from build123d import *

# Parameters (mm, degrees)
F0_R     = 10.5
F0_R_2   = 9.5
F1_DEPTH = 10
F0_W     = 35
F0_H     = 35
F2_DEPTH = 1
F3_R     = 0.4
F4_R     = 0.5


with BuildPart() as f1:
    # F0 (on Top) → F1 (new body)
    with BuildSketch(Plane.XY):
        Circle(F0_R)
        Circle(F0_R_2, mode=Mode.SUBTRACT)
    extrude(amount=F1_DEPTH)

    # F0 (on Top) → F2 (join)
    with BuildSketch(Plane.XY):
        Rectangle(F0_W, F0_H)
        Circle(F0_R, mode=Mode.SUBTRACT)
        Circle(F0_R)
        Circle(F0_R_2, mode=Mode.SUBTRACT)
        Circle(F0_R_2)
    extrude(amount=-F2_DEPTH)

    # F3
    f3_edges = [f1.edges().sort_by_distance(p)[0] for p in [
        (-17.5, 0, -1),
        (0, 17.5, -1),
        (17.5, 0, -1),
        (0, -17.5, -1),
    ]]
    fillet(f3_edges, radius=F3_R)

    # F4
    f4_edges = [f1.edges().sort_by_distance(p)[0] for p in [
        (-9.5, 0, 10),
    ]]
    fillet(f4_edges, radius=F4_R)


solid = f1.part
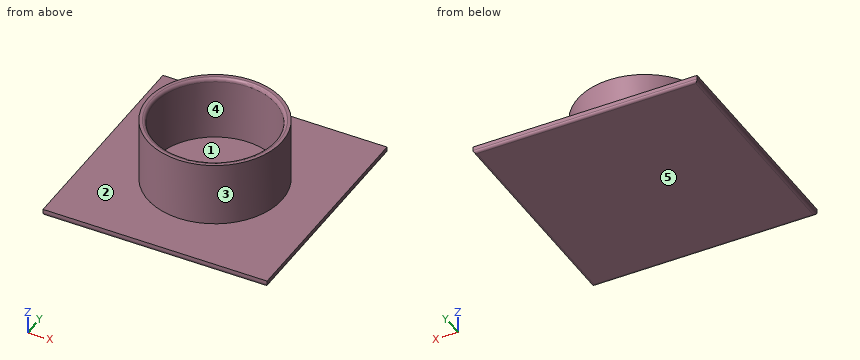
Check sheet for the modelled part. Datum: model origin and axes. Units: mm. Face numbers are marked on the shaded views. A direction names the side the tool comes from. Give positions to 0.01 mm unless a question says otherwise; leave off trailing zeros. Order: outer loops, then holes, each group sorted by start corner. A loop starts at its lowest first (then second) coordinate and runs counter-clockwise, first axis right, second up. Notation, with made-up numbers: M 64,-1 L 84,-1 A7 cw 84,6 Z; hole C -5,63 d4. An arc over 180 degrees is marked long. Answer as CSV lines item,"result". Start each with the question number.
Item 1: Cross-section at D-D on x = 12.5. Enter the section's corners in (y, z).
Item 2: Mould release check, pull along X, two halves, no side actions. Record for the marked faces 1, 2 and 3: +X half, -X half, draft (parallel to the pull), parting line (faces both ways), or undercut.
Item 3: Gauge pin test, flat ends, axial feed: P1, Ø3, axis at y = -4.5, z = 5.5, coming from the -X side; P2, Ø5.5, axis at x = 4, y = 1, coming from the +Z side; P3, Ø4, axis at y = 4.5, z = 5.5, coming from the +X side. Record the tip position at first contact, or that the pin passes through.
Item 4: Cross-section at A-A on y = 0. Enter the section's corners in (x, z).
Item 5: Cross-section at C-C on z = 4. Enter the section's corners in (x, y).
Item 6: Tool access check on the marked faces 4 and 5. Record the directions out of +Z, -Z, +X, -X, +Y, -Y that give a thin tool (end or side, any length) a straight path to the whole face; none if there is none.
Item 7: Thickness scan on line 1 (Y direction, x = 0, z = 5); line 2 (Z direction, x = -5, y = 7.5); line 3 (X direction, y = 4.5, z = 3.75). Record the ranges inside material, lowest first. Write a range as [from, to].
Established:
1,outline,"M -17.5,-0.6 A0.4 ccw -17.1,-1 L 17.1,-1 A0.4 ccw 17.5,-0.6 L 17.5,0 L -17.5,0 Z"
2,face 1,"undercut"
2,face 2,"draft"
2,face 3,"parting line"
3,P1,"stops at x = -10.06"
3,P2,"stops at z = 0"
3,P3,"stops at x = 10.2"
4,outline,"M -17.5,-0.6 A0.4 ccw -17.1,-1 L 17.1,-1 A0.4 ccw 17.5,-0.6 L 17.5,0 L 10.5,0 L 10.5,10 L 10,10 A0.5 ccw 9.5,9.5 L 9.5,0 L -9.5,0 L -9.5,9.5 A0.5 ccw -10,10 L -10.5,10 L -10.5,0 L -17.5,0 Z"
5,outline,"C 0,0 d21; hole C 0,0 d19"
6,face 4,"+Z"
6,face 5,"-Z, +X, -X, +Y, -Y"
7,line 1,"y = [-10.5, -9.5], [9.5, 10.5]"
7,line 2,"z = [-1, 0]"
7,line 3,"x = [-9.49, -8.37], [8.37, 9.49]"
